from build123d import *

# Parameters (mm, degrees)
SKETCH_R      = 4
PAD_DEPTH     = 4
SKETCH001_R   = 6.5
SKETCH001_R_2 = 4
PAD001_DEPTH  = 4.8
CHAMFER_SIZE  = 0.5
FILLET_R      = 3


with BuildPart() as part:
    # Sketch → Pad (new body)
    with BuildSketch(Plane.XY):
        Polygon((0, 16.36788), (-14.175, 8.18394), (-14.175, -8.18394), (0, -16.36788), (14.175, -8.18394), (14.175, 8.18394), align=None)
        Circle(SKETCH_R, mode=Mode.SUBTRACT)
    extrude(amount=PAD_DEPTH)

    # Sketch001 (on Face9 of Pad) → Pad001 (join)
    with BuildSketch(Plane.XY.offset(4)):
        Circle(SKETCH001_R)
        Circle(SKETCH001_R_2, mode=Mode.SUBTRACT)
    extrude(amount=PAD001_DEPTH)

    # Chamfer
    chamfer_edges = [part.edges().sort_by_distance(p)[0] for p in [
        (-4, 0, 8.8),
    ]]
    chamfer(chamfer_edges, length=CHAMFER_SIZE)

    # Fillet
    fillet_edges = [part.edges().sort_by_distance(p)[0] for p in [
        (0, -16.36788, 2),
        (14.175, -8.18394, 2),
        (14.175, 8.18394, 2),
        (-14.175, -8.18394, 2),
        (-14.175, 8.18394, 2),
        (0, 16.36788, 2),
    ]]
    fillet(fillet_edges, radius=FILLET_R)


solid = part.part
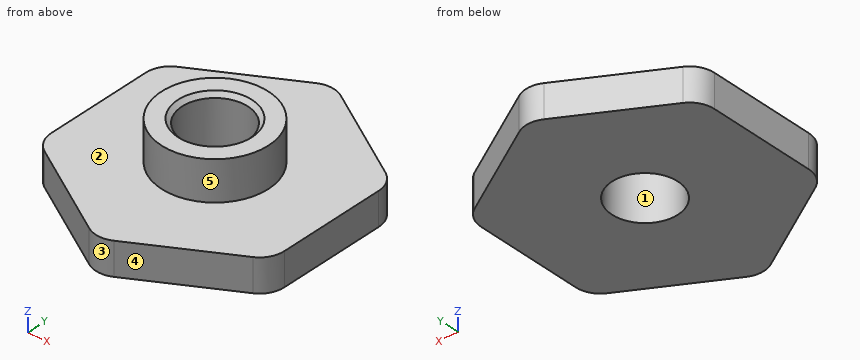
Geometry check sheet. Reference: the model listing, model coordinates, mm. Face numbers are marked on the shaded views. A direction names the side the tool comes from. Give positions to 0.01 mm unless a question says otherwise; leave off trailing zeros. Write each loop counter-clockwise with the first axis right and the second up, starting at its lowest first coordinate (ties: lowest second). Pieces come first, ordered by that corner, then holes. Notation, with made-up numbers: M 71,23.5 L 83,23.5 A14 cw 83,48.5 Z; hole C 35.25,85.25 d1. An arc over 180 degrees is marked long. Answer as CSV lines item,"result". Start each with the question number.
Q1. Tool access check on the marked faces 4 and 5. Record the directions out of +Z, -Z, +X, -X, +Y, -Y that give a thin tool (end or side, any length) a straight path to the whole face; none if there is none.
Q2. Section check D-D, the plane x = -5.75. Record the cut outline in (y, z).
Q3. Release check for a two-part mould opening along X. For the marked faces 1, 2 and 3 record: pulls with the +X half, pulls with the -X half, needs draft (parallel to the pull), parting line crosses it, or undercut.
Q4. Section check A-A, the plane y = 0. Record the cut outline in (x, z) (3 decimals).
Q5. Go/stop test with flat-tipped pins: pin 1 (12 mm diameter, centred on x = 1, y = 1, fed in from +Z); pin 2 (5 mm diameter, centred on x = 0, y = 0, fed in from -Z); pin 3 (2 mm diameter, centred on x = -11, z = 2.5, fed in from +Y); pin 4 (1.5 mm diameter, centred on x = 9, z = 4, fed in from +Y). Record where each tip stops, or that it passes through.
Q6. Material ranges on L1, parallel to Y at x = 0, z = 4.5; L2, parallel to Z at x = 0, y = 8; L3, parallel to Y at x = 0, z = 2, recorded low to high.
Q7. Section check C-C, the plane x = 0. Record the cut outline in (y, z).
Q8. Section check B-B, the plane z = 2.75. Record the cut outline in (x, y) (3 decimals).
Geometry says:
1,face 4,"+Z, -Z, +X, -Y"
1,face 5,"+Z"
2,outline,"M -13.05,0 L 13.05,0 L 13.05,4 L 3.03,4 L 3.03,8.8 L -3.03,8.8 L -3.03,4 L -13.05,4 Z"
3,face 1,"undercut"
3,face 2,"needs draft"
3,face 3,"parting line crosses it"
4,outline,"M -14.175,0 L -4,0 L -4,8.3 L -4.5,8.8 L -6.5,8.8 L -6.5,4 L -14.175,4 Z; M 4,0 L 14.175,0 L 14.175,4 L 6.5,4 L 6.5,8.8 L 4.5,8.8 L 4,8.3 Z"
5,pin 1,"z = 8.8"
5,pin 2,"through"
5,pin 3,"y = 10.59"
5,pin 4,"y = 11.6"
6,L1,"-6.5 to -4, 4 to 6.5"
6,L2,"0 to 4"
6,L3,"-15.9 to -4, 4 to 15.9"
7,outline,"M -15.9,0 L -4,0 L -4,8.3 L -4.5,8.8 L -6.5,8.8 L -6.5,4 L -15.9,4 Z; M 4,0 L 15.9,0 L 15.9,4 L 6.5,4 L 6.5,8.8 L 4.5,8.8 L 4,8.3 Z"
8,outline,"M -14.175,-6.452 A3 ccw -12.675,-9.05 L -1.5,-15.502 A3 ccw 1.5,-15.502 L 12.675,-9.05 A3 ccw 14.175,-6.452 L 14.175,6.452 A3 ccw 12.675,9.05 L 1.5,15.502 A3 ccw -1.5,15.502 L -12.675,9.05 A3 ccw -14.175,6.452 Z; hole C 0,0 d8"
